from build123d import *

# Parameters (mm, degrees)
SKETCH1_W           = 120
SKETCH1_H           = 100
SKETCH1_R           = 2.5
BOSS_EXTRUDE1_DEPTH = 5
SKETCH2_R           = 2.5
BOSS_EXTRUDE2_DEPTH = 45
CHAMFER1_SIZE       = 1
SKETCH3_W           = 120
SKETCH3_H           = 100
SKETCH3_W_2         = 40
SKETCH3_H_2         = 40
CUT_EXTRUDE1_DEPTH  = 2.5
SKETCH6_W           = 15
SKETCH6_H           = 40
CUT_EXTRUDE2_DEPTH  = 89.917096219
FILLET1_R           = 2
FILLET2_R           = 2


with BuildPart() as part:
    # Sketch1 → Boss-Extrude1 (new body)
    with BuildSketch(Plane.XY):
        Rectangle(SKETCH1_W, SKETCH1_H)
        Circle(SKETCH1_R, mode=Mode.SUBTRACT)
    extrude(amount=BOSS_EXTRUDE1_DEPTH)

    # Sketch2 → Boss-Extrude2 (add)
    with BuildSketch(Plane.XY):
        with Locations(Location((0, 0, 0), (0, 0, 180))):
            Circle(SKETCH2_R)
    extrude(amount=BOSS_EXTRUDE2_DEPTH)

    # Chamfer1
    chamfer1_edges = [part.edges().sort_by_distance(p)[0] for p in [
        (2.5, 0, 45),
    ]]
    chamfer(chamfer1_edges, length=CHAMFER1_SIZE)

    # Sketch3 → Cut-Extrude1 (cut)
    with BuildSketch(Plane.XY.offset(5)):
        Rectangle(SKETCH3_W, SKETCH3_H)
        Rectangle(SKETCH3_W_2, SKETCH3_H_2, mode=Mode.SUBTRACT)
    extrude(amount=-CUT_EXTRUDE1_DEPTH, mode=Mode.SUBTRACT)

    # Sketch6 → Cut-Extrude2 (cut, through all)
    with BuildSketch(Plane.XY.offset(2.5)):
        with Locations((-27.5, 0)):
            Rectangle(SKETCH6_W, SKETCH6_H)
        with Locations((27.5, 0)):
            Rectangle(SKETCH6_W, SKETCH6_H)
    extrude(amount=-CUT_EXTRUDE2_DEPTH, mode=Mode.SUBTRACT)

    # Fillet1
    fillet1_edges = [part.edges().sort_by_distance(p)[0] for p in [
        (60, -50, 1.25),
        (-60, -50, 1.25),
        (-60, 50, 1.25),
        (60, 50, 1.25),
        (60, 0, 2.5),
        (0, -50, 2.5),
        (-60, 0, 2.5),
        (0, 50, 2.5),
    ]]
    fillet(fillet1_edges, radius=FILLET1_R)

    # Fillet2
    fillet2_edges = [part.edges().sort_by_distance(p)[0] for p in [
        (-35, -20, 1.25),
        (-35, 20, 1.25),
        (35, 20, 1.25),
        (35, -20, 1.25),
    ]]
    fillet(fillet2_edges, radius=FILLET2_R)


solid = part.part
Check sheet for the modelled part. Datum: model origin and axes. Units: mm. A direction names the side the tool comes from. Round coordinates to 2 decimals unless told otherwise and drop trailing zeros. Order: outer loops, then holes, each group sorted by start corner. A loop starts at its lowest first (then second) coordinate and runs counter-clockwise, first axis right, second up.
(1) Cross-section at D-D, the plane y = -29. Enter the section's corners in (x, z).
(2) Scan lines: probe 1 along Z at (x, y) = (-4.5, 32); probe 2 along Z at (x, y) = (3, 8). Record each from-to range of solid material in increasing order.
(3) Go/stop test with flat-tipped pins: P1, Ø8, axis at x = 43.5, y = 39, coming from the +Z side; P2, Ø0.8, axis at y = 1.5, z = 1.5, coming from the +X side; P3, Ø1.2, axis at x = -5.5, z = 3.5, coming from the +Y side. Record where each tip stops, or that it passes through.
(4) Cross-section at B-B, the plane x = -30. Enter the section's corners in (y, z), and give its area (3 significant figures).
(5) Cross-section at C-C, the plane x = -15. Enter the section's corners in (y, z), and give its area (3 significant figures).
(6) Access from +Z, -Z, +X, -X, +Y, -Y to the whole of each face (thin tool, end or side, straight path). Record for faces 1 (the flat face through (26, 20, 1)), 2 (the flat face through (0, 20, 4)), 3 (the cylindrical face through (2.5, -0.1, 24.2)), 4 (the flat face through (0, -20, 4)), 5 (the flat face through (0, 0, 45)).
(7) Cross-section at A-A, the plane y = 8.5. Enter the section's corners in (x, z).
Check sheet entries:
1. outline: (-60, 0) - (60, 0) - (60, 0.5) arc R2 ccw to (58, 2.5) - (-58, 2.5) arc R2 ccw to (-60, 0.5) - close
2. probe 1: z = 0 to 2.5
2. probe 2: z = 0 to 5
3. P1: stops at z = 2.5
3. P2: stops at x = 59.91
3. P3: stops at y = 20
4. outline: (-50, 0) - (-20, 0) - (-20, 2.5) - (-48, 2.5) arc R2 ccw to (-50, 0.5) - close; (20, 0) - (50, 0) - (50, 0.5) arc R2 ccw to (48, 2.5) - (20, 2.5) - close
4. area: 148 mm2
5. outline: (-50, 0) - (50, 0) - (50, 0.5) arc R2 ccw to (48, 2.5) - (20, 2.5) - (20, 5) - (-20, 5) - (-20, 2.5) - (-48, 2.5) arc R2 ccw to (-50, 0.5) - close
5. area: 348 mm2
6. face 1: +Z, -Z
6. face 2: +Z, +X, -X, +Y
6. face 3: +Z
6. face 4: +Z, +X, -X, -Y
6. face 5: +Z, +X, -X, +Y, -Y
7. outline: (-60, 0) - (-35, 0) - (-35, 2.5) - (-58, 2.5) arc R2 ccw to (-60, 0.5) - close; (-20, 0) - (20, 0) - (20, 5) - (-20, 5) - close; (35, 0) - (60, 0) - (60, 0.5) arc R2 ccw to (58, 2.5) - (35, 2.5) - close
